Here's the drawing with two shaded views (mm, measured from the low corner). I have some questions. Give positions to 0.01 mm unless a question says otherwise; leave off trailing zeros. Order: outer loops, then holes, each group sorted by start corner. A loop starts at its lowest first (then second) coordinate and runs counter-clockwise, first axis right, second up. Notation, with made-up numbers: (21.5, -6.5) - (75.5, -6.5) arc R26 cw to (75.5, 27.5) - close; hole circle Ø8 at (50, 41.5). An arc over 180 degrees is marked (long way). Use one line per item in the form item = value. Start each with the question number.
1) Please list where these lines run through material, in increasing order: probe 1 along X at (y, z) = (10.1, 55) (3 decimals); probe 2 along X at (y, z) = (9, 15); probe 3 along Z at (x, y) = (21, 9.75).
2) Suppose I cut it at B-B, the plane x = 11. Write out the boundary of the cut face in (y, z).
3) Suppose I cut it at A-A, the plane z = 24.5. Write out the boundary of the cut face in (x, y).
4) For pin 1 (3 mm diameter, centred on x = 26.725, z = 55, fed in from +Y); pin 2 (8 mm diameter, centred on x = 14.5, z = 12, fed in from -Y); pin 3 (6.5 mm diameter, centred on x = 17.075, z = 5, fed in from +Y), each with a flat end and sliding along its axis, tell me the tip position at first contact or that it passes through.
5) Suppose I cut it at C-C, the plane z = 5. Write out the boundary of the cut face in (x, y) (3 decimals).
6) We'd pull the mould along Z, two halves only. Please class the marked faces 1, 2 and 3: released by +Z, released by -Z, zero draft, split by the parting line, or undercut.
7) Suppose I cut it at D-D, the plane y = 5.5. Write out the boundary of the cut face in (x, z).
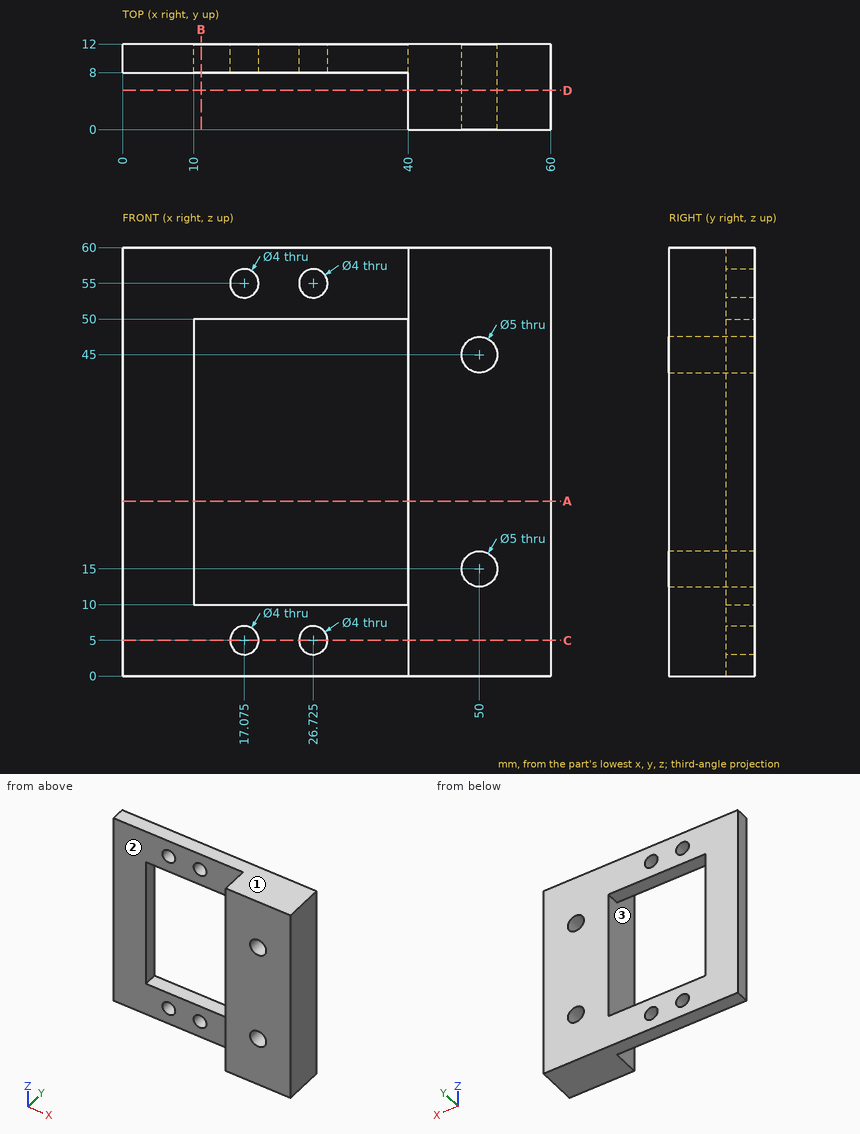
Result sheet:
q1.probe_1 = 0 to 15.075, 19.075 to 24.725, 28.725 to 60
q1.probe_2 = 0 to 10, 40 to 47.5, 52.5 to 60
q1.probe_3 = 0 to 10, 50 to 60
q2.outline = (8, 0) - (12, 0) - (12, 10) - (8, 10) - close; (8, 50) - (12, 50) - (12, 60) - (8, 60) - close
q3.outline = (0, 8) - (10, 8) - (10, 12) - (0, 12) - close; (40, 0) - (60, 0) - (60, 12) - (40, 12) - close
q4.pin_1 = through
q4.pin_2 = 8
q4.pin_3 = 12
q5.outline = (0, 8) - (15.075, 8) - (15.075, 12) - (0, 12) - close; (19.075, 8) - (24.725, 8) - (24.725, 12) - (19.075, 12) - close; (28.725, 8) - (40, 8) - (40, 0) - (60, 0) - (60, 12) - (28.725, 12) - close
q6.face_1 = released by +Z
q6.face_2 = zero draft
q6.face_3 = undercut
q7.outline = (40, 0) - (60, 0) - (60, 60) - (40, 60) - close; hole circle Ø5 at (50, 15); hole circle Ø5 at (50, 45)
